Autodesk Inventor part; units mm, degrees
ref_plane "Work Plane1" through (-19.6075, -25, -15) normal (0, 0, 1) x (1, 0, 0)
ref_plane "Work Plane2" through (-137.3725, -100, -40) normal (0, 0, -1) x (0, 1, 0)
ref_plane "Work Plane3" through (-19.6075, -25, -15) normal (0, 0, 1) x (1, 0, 0)
sketch "Sketch1" plane through (0, 0, 0) normal (0, 0, 1) x (1, 0, 0)
  circle A0 centre (0, 0) radius 19.4
  circle A1 centre (0, 0) radius 14
  dimension "d0" = 38.8
  dimension "d1" = 28
extrude "Extrusion1" add sketch "Sketch1" against normal blind 2
ref_plane "Work Plane1" through (-19.6075, -25, -15) normal (0, 0, 1) x (1, 0, 0)
ref_plane "Work Plane2" through (-137.3725, -100, -40) normal (0, 0, -1) x (0, 1, 0)
sketch "Sketch5" plane through (0, 0, -2) normal (0, 0, -1) x (-1, 0, 0)
  circle A0 centre (0, 0) radius 19.4
  line L0 (-5.456, -3.15) -> (-5.456, 3.15)
  line L1 (-5.456, 3.15) -> (0, 6.3)
  line L2 (0, 6.3) -> (5.456, 3.15)
  line L3 (5.456, 3.15) -> (5.456, -3.15)
  line L4 (5.456, -3.15) -> (0, -6.3)
  line L5 (0, -6.3) -> (-5.456, -3.15)
  dimension "d14" = 6.3
extrude "Extrusion5" add sketch "Sketch5" along normal blind 3
sketch "Sketch6" plane through (0, 0, -5) normal (0, 0, -1) x (-1, 0, 0)
  circle A0 centre (0, 0) radius 19.4
  line L0 (-5.456, -3.15) -> (-5.456, 3.15)
  line L1 (-5.456, 3.15) -> (0, 6.3)
  line L2 (0, 6.3) -> (5.456, 3.15)
  line L3 (5.456, 3.15) -> (5.456, -3.15)
  line L4 (5.456, -3.15) -> (0, -6.3)
  line L5 (0, -6.3) -> (-5.456, -3.15)
  line L6 (-6.456, 3.7274) -> (-6.456, -3.7274)
  line L7 (-6.456, -3.7274) -> (0, -7.4547)
  line L8 (0, -7.4547) -> (6.456, -3.7274)
  line L9 (6.456, -3.7274) -> (6.456, 3.7274)
  line L10 (6.456, 3.7274) -> (0, 7.4547)
  line L11 (0, 7.4547) -> (-6.456, 3.7274)
  dimension "d17" = 1
ref_plane "Work Plane3" through (-19.6075, -25, -15) normal (0, 0, 1) x (1, 0, 0)
extrude "Extrusion6" add sketch "Sketch6" along normal up to surface (10 mm away) contours L0 L1 L2 L3 L4 L5 | L11 L10 L9 L8 L7 L6
sketch "Sketch7" plane through (6.456, -3.7274, -15) normal (0, 0, -1) x (-1, 0, 0)
  circle A0 centre (6.456, 3.7274) radius 4
  dimension "d20" = 8
ref_plane "Work Plane4" through (-137.3725, -100, -40) normal (0, 0, -1) x (0, 1, 0)
extrude "Extrusion7" add sketch "Sketch7" along normal up to surface (25 mm away)
sketch "Sketch8" plane through (0, 0, -40) normal (0, 0, -1) x (-1, 0, 0)
  line L0 (-3, -1) -> (3, -1)
  line L1 (3, -1) -> (3, 1)
  line L2 (3, 1) -> (-3, 1)
  line L3 (-3, 1) -> (-3, -1)
  line L4 (-3, -1) -> (3, 1) construction
  line L5 (3, -1) -> (-3, 1) construction
  point P0 (0, 0)
  dimension "d23" = 6
  dimension "d24" = 2
extrude "Extrusion8" add sketch "Sketch8" along normal blind 10
thicken "Thicken1" operation cut thickness 0.4 both sides no extend neighbours no toward (0.9870503, 0.1604113, 0) faces at (-3.9482, -0.6416, -31.6667)
thicken "Thicken2" operation cut thickness 0.4 both sides no extend neighbours no toward (1, 0, 0) faces at (-3, -0.3333, -46.6667) (-1, 1, -43.3333) (3, 0.3333, -46.6667) (1, -1, -43.3333) (-1, -0.3333, -50)
properties part number "Reverser_print"
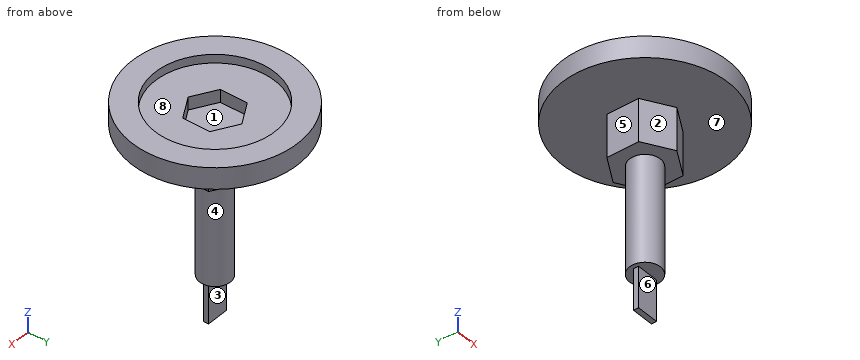
Verification items for the finished model (mm, model axes). Face numbers are marked on the shaded views. A direction names the side the tool comes from. Coordinates: 2 decimals unless noted, no trailing zeros. Loops run counter-clockwise (first coordinate to the right, second up) from the corner with the lowest first, then second, coordinate; pieces in that order, holes last. Notation, with made-up numbers: (23.5, 88.25) -> (49.5, 88.25) arc R15 ccw to (49.5, 114.25) -> close; hole circle Ø7 at (36.25, -39). An arc over 180 degrees is marked (long way). Put each result on its own line as item: value.
1. Section check B-B, the plane x = 7.5. Record the boundary of the cut face in (y, z), then the cut area to 3 significant figures.
Result set:
outline: (-17.89, -5) -> (17.89, -5) -> (17.89, 0) -> (11.82, 0) -> (11.82, -2) -> (-11.82, -2) -> (-11.82, 0) -> (-17.89, 0) -> close
area: 132 mm^2
2. Thickness scan on line 1 (Y direction, x = 0, z = -1); line 2 (Z direction, x = 13, y = -2); line 3 (Z direction, x = -13, y = 6.5). Record the ranges inside material, lowest first.
Result set:
line 1: y = -19.4 to -14, 14 to 19.4
line 2: z = -5 to -2
line 3: z = -5 to 0
3. Mould release check, pull along X, two halves, no side actions. Record for the marked faces 1, 2, 3 and 4: pulls with the +X half, pulls with the -X half, needs draft (parallel to the pull), parting line crosses it, or undercut.
Result set:
face 1: undercut
face 2: pulls with the -X half
face 3: needs draft
face 4: parting line crosses it
4. Section check A-A, the plane z = -3.5. Record the boundary of the cut face in (x, y), then the cut area to 3 significant figures.
Result set:
outline: circle Ø38.8 at (0, 0); hole (-5.46, -3.15) -> (0, -6.3) -> (5.46, -3.15) -> (5.46, 3.15) -> (0, 6.3) -> (-5.46, 3.15) -> close
area: 1,080 mm^2
5. Gauge pin test, flat ends, axial feed: P1, Ø8.5, axis at x = 1, y = -1, coming from the +Z side; P2, Ø1, axis at y = 1, z = -8.5, coming from the +X side; P3, Ø1.6, axis at x = -0.5, z = -44, coming from the +Y side; P4, Ø2, axis at y = 10, z = -9, coming from the +X side. Record the tip position at first contact, or that the pin passes through.
Result set:
P1: stops at z = -2
P2: stops at x = 6.46
P3: stops at y = 0.6
P4: passes through
6. Section check C-C, the plane y = 0. Record the boundary of the cut face in (x, z), then the cut area to 3 significant figures.
Result set:
outline: (-19.4, -5) -> (-6.46, -5) -> (-6.46, -15) -> (-3.6, -15) -> (-3.6, -40) -> (-2.6, -40) -> (-2.6, -49.6) -> (2.6, -49.6) -> (2.6, -40) -> (3.6, -40) -> (3.6, -15) -> (6.46, -15) -> (6.46, -5) -> (19.4, -5) -> (19.4, 0) -> (14, 0) -> (14, -2) -> (5.46, -2) -> (5.46, -5) -> (-5.46, -5) -> (-5.46, -2) -> (-14, -2) -> (-14, 0) -> (-19.4, 0) -> close
area: 464 mm^2
7. Tool access check on the marked faces 5, 6, 7 and 8. Record the directions out of +Z, -Z, +X, -X, +Y, -Y that give a thin tool (end or side, any length) a straight path to the whole face; none if there is none.
Result set:
face 5: -Z, -X, +Y, -Y
face 6: -Z, +X, -X, -Y
face 7: -Z
face 8: +Z
8. Section check D-D, the plane z = -42. Record the boundary of the cut face in (x, y).
Result set:
outline: (-2.6, -0.6) -> (2.6, -0.6) -> (2.6, 0.6) -> (-2.6, 0.6) -> close
